from build123d import *

# Parameters (mm, degrees)
SKETCH_W        = 4.72
SKETCH_H        = 5.2
PAD_DEPTH       = 18.3
POCKET_DEPTH    = 38.001
SKETCH002_R     = 1.5
POCKET001_DEPTH = 6
PAD001_DEPTH    = 13
SKETCH004_W     = 2
SKETCH004_H     = 0.982872
POCKET002_DEPTH = 38.001
POCKET003_DEPTH = 51.701
FILLET_R        = 1
CHAMFER_SIZE    = 0.5
FILLET001_R     = 1


with BuildPart() as part:
    # Sketch → Pad (new body)
    with BuildSketch(Plane.XY):
        Polygon((-19, 22), (-19, -22), (19, -22), (19, 22), (17, 22), (17, 29.7), (6, 29.7), (6, 22), (-6, 22), (-6, 29.7), (-17, 29.7), (-17, 22), align=None)
        with Locations((-12.41, 24.6)):
            Rectangle(SKETCH_W, SKETCH_H, mode=Mode.SUBTRACT)
        with Locations((12.41, 24.6)):
            Rectangle(SKETCH_W, SKETCH_H, mode=Mode.SUBTRACT)
    extrude(amount=PAD_DEPTH)

    # Sketch001 (on Face3 of Pad) → Pocket (cut, through all)
    with BuildSketch(Plane.YZ.offset(19)):
        with BuildLine():
            Line((29.7, 11.3), (29.7, 0))
            Line((29.7, 0), (-21.3, 0))
            ThreePointArc((3.7, 11.3), (-10.017598, 8.343801), (-21.3, 0))
            Line((29.7, 11.3), (3.7, 11.3))
        make_face()
    extrude(amount=-POCKET_DEPTH, mode=Mode.SUBTRACT)

    # Sketch002 (on Face5 of Pocket) → Pocket001 (cut)
    with BuildSketch(Plane.XZ.offset(22)):
        with Locations((-15.844609, 11.767382)):
            Circle(SKETCH002_R)
        with Locations((15.754541, 11.777902)):
            Circle(SKETCH002_R)
    extrude(amount=-POCKET001_DEPTH, mode=Mode.SUBTRACT)

    # Sketch003 (on Face1 of Pocket001) → Pad001 (join)
    with BuildSketch(Plane(origin=(-19, 0, 0), x_dir=(0, -1, 0), z_dir=(-1, 0, 0))):
        with BuildLine():
            Line((20, 18.3), (1.881002, 18.3))
            ThreePointArc((1.881002, 18.3), (10.537629, 21.219302), (15.5, 28.88966))
            Line((20, 28.88966), (15.5, 28.88966))
            Line((20, 18.3), (20, 28.88966))
        make_face()
    pad001 = extrude(amount=-PAD001_DEPTH)

    # Mirrored: Pad001 across YZ
    add(pad001.mirror(Plane.YZ))

    # Sketch004 (on Face5 of Mirrored) → Pocket002 (cut, through all)
    with BuildSketch(Plane(origin=(-19, 0, 0), x_dir=(0, -1, 0), z_dir=(-1, 0, 0))):
        with Locations((21, 17.808564)):
            Rectangle(SKETCH004_W, SKETCH004_H)
    extrude(amount=-POCKET002_DEPTH, mode=Mode.SUBTRACT)

    # Sketch005 (on Face23 of Pocket002) → Pocket003 (cut, through all)
    with BuildSketch(Plane.XZ.offset(22)):
        with BuildLine():
            add(Edge.make_bspline(
                [(-19.030813, 9.913328), (-19.030294, 8.01238), (-17.308198, 7.207429)],
                knots=[1.082896, 1.082896, 1.082896, 2.216203, 2.216203, 2.216203], degree=2, weights=[1, 0.843702, 1]))
            Line((-17.308198, 7.207429), (-3.577259, 0.790051))
            add(Edge.make_bspline(
                [(-3.577259, 0.790051), (-1.968517, 0.037468), (-0.192474, 0.03938)],
                knots=[2.215888, 2.215888, 2.215888, 2.654527, 2.654527, 2.654527], degree=2, weights=[1, 0.976046, 1]))
            Line((-0.192474, 0.03938), (0.111534, 0.039482))
            add(Edge.make_bspline(
                [(0.111534, 0.039482), (1.887576, 0.038752), (3.495769, 0.792404)],
                knots=[2.653039, 2.653039, 2.653039, 3.091677, 3.091677, 3.091677], degree=2, weights=[1, 0.976046, 1]))
            Line((3.495769, 0.792404), (17.222042, 7.218925))
            add(Edge.make_bspline(
                [(17.222042, 7.218925), (18.943553, 8.025023), (18.94269, 9.92597)],
                knots=[3.091363, 3.091363, 3.091363, 4.22467, 4.22467, 4.22467], degree=2, weights=[1, 0.843702, 1]))
            Line((18.94269, 9.92597), (19.755945, 10.17424))
            Line((19.755945, 10.17424), (19.755945, -1.191288))
            Line((19.755945, -1.191288), (-20.023405, -1.191288))
            Line((-20.023405, -1.191288), (-20.023405, 9.913328))
            Line((-20.023405, 9.913328), (-19.030813, 9.913328))
        make_face()
    extrude(amount=-POCKET003_DEPTH, mode=Mode.SUBTRACT)

    # Fillet
    fillet_edges = [part.edges().sort_by_distance(p)[0] for p in [
        (19, 22, 14.8),
        (17, 29.7, 14.8),
        (6, 29.7, 14.8),
        (-6, 29.7, 14.8),
        (-17, 29.7, 14.8),
        (-19, 22, 14.8),
    ]]
    fillet(fillet_edges, radius=FILLET_R)

    # Chamfer
    chamfer_edges = [part.edges().sort_by_distance(p)[0] for p in [
        (12.41, 22, 11.3),
        (10.05, 24.6, 11.3),
        (12.41, 27.2, 11.3),
        (14.77, 24.6, 11.3),
        (-10.05, 24.6, 11.3),
        (-12.41, 22, 11.3),
        (-14.77, 24.6, 11.3),
        (-12.41, 27.2, 11.3),
    ]]
    chamfer(chamfer_edges, length=CHAMFER_SIZE)

    # Fillet001
    fillet001_edges = [part.edges().sort_by_distance(p)[0] for p in [
        (-12.5, -15.5, 28.88966),
        (12.5, -15.5, 28.88966),
    ]]
    fillet(fillet001_edges, radius=FILLET001_R)


solid = part.part
Read the model definition and answer for the solid it produces. Units are mm, in the model's axes. A direction names the side the tool comes from. Round coordinates to 2 decimals unless told otherwise and drop trailing zeros. Write each loop counter-clockwise with the first axis right and the second up, starting at its lowest first coordinate (ties: lowest second). Pieces come first, ordered by that corner, then holes. Notation, with made-up numbers: M 15.5,-21 L 71.5,-21 A17 ccw 71.5,-14 Z; hole C 22,-28 d10. An arc over 180 degrees is marked long. Use a Markdown table: item, result.
1) A tool of negligible diameter and unlimited length cuts with its end or side. For faces 4 (the flat face through (6, 25, 15)), 5 (the flat face through (-12, 27.2, 15)), 6 (the flat face through (-6, -15, 22)), from which of +Z, -Z, +X, -X, +Y, -Y can it reach the whole face along a straight path? Write none if from no direction.
Answers follow:
| item | result |
|---|---|
| face 4 | +Z, -Z, +Y |
| face 5 | +Z, -Z |
| face 6 | +Z, +Y, -Y |
2) The part is cut by section C-C (x = -12). Write down the section's boundary in (y, z).
Answers follow:
| item | result |
|---|---|
| outline | M -22,4.73 L -16.17,4.73 A33.3 cw 3.7,11.3 L 21.5,11.3 L 22,11.8 L 22,18.3 L -2.17,18.3 A13.87 cw -15.31,28.18 A1 ccw -16.26,28.89 L -20,28.89 L -20,17.32 L -22,17.32 Z; M 27.2,11.8 L 27.7,11.3 L 29.7,11.3 L 29.7,18.3 L 27.2,18.3 Z |
3) The part is cut by section A-A (y = 25). Write down the section's boundary in (x, z), plus the area to 3 significant figures.
Answers follow:
| item | result |
|---|---|
| outline | M -17,11.3 L -15.27,11.3 L -14.77,11.8 L -14.77,18.3 L -17,18.3 Z; M -10.05,11.8 L -9.55,11.3 L -6,11.3 L -6,18.3 L -10.05,18.3 Z; M 6,11.3 L 9.55,11.3 L 10.05,11.8 L 10.05,18.3 L 6,18.3 Z; M 14.77,11.8 L 15.27,11.3 L 17,11.3 L 17,18.3 L 14.77,18.3 Z |
| area | 87.4 mm2 |
4) Straight lines are drawn through the part: line 1 along X through (y, z) = (-7.5, 19.25); line 2 along Z through (x, y) = (3, -4.5); line 3 along Z through (x, y) = (8, 19). For each, find the intervals that lie inside material, in ascending order. Write a range as [from, to].
Answers follow:
| item | result |
|---|---|
| line 1 | x = [-19, -6], [6, 19] |
| line 2 | z = [10.27, 18.3] |
| line 3 | z = [11.3, 18.3] |
5) The part is cut by section B-B (z = 16.25). Write down the section's boundary in (x, y), plus the area to 3 significant figures.
Answers follow:
| item | result |
|---|---|
| outline | M -19,-22 L 19,-22 L 19,21 A1 ccw 18,22 L 17,22 L 17,28.7 A1 ccw 16,29.7 L 7,29.7 A1 ccw 6,28.7 L 6,22 L -6,22 L -6,28.7 A1 ccw -7,29.7 L -16,29.7 A1 ccw -17,28.7 L -17,22 L -18,22 A1 ccw -19,21 Z; hole M -14.77,22 L -10.05,22 L -10.05,27.2 L -14.77,27.2 Z; hole M 10.05,22 L 14.77,22 L 14.77,27.2 L 10.05,27.2 Z |
| area | 1,790 mm2 |
6) For a pull along X with two mould halves and no side action, classify faces 1 (the flat face through (12, 22, 15)), 2 (the flat face through (-12.065, -19.372, 4.757)), 3 (the flat face through (-13, -18, 28.89)) as pulls with the +X half, pulls with the -X half, needs draft (parallel to the pull), parting line crosses it, or undercut.
Answers follow:
| item | result |
|---|---|
| face 1 | undercut |
| face 2 | pulls with the -X half |
| face 3 | needs draft |
7) Flat-ended cylindrical pins translate along their axes: pin 1 (4 mm diameter, centred on y = 26, z = 14, fed in from -X); pin 2 (4 mm diameter, centred on x = 11, y = -10.5, fed in from -Z); pin 3 (8 mm diameter, centred on x = 7, y = -14.5, fed in from -Z). Find the tip coordinate at first contact, or state that the pin passes through.
Answers follow:
| item | result |
|---|---|
| pin 1 | stops at x = -17 |
| pin 2 | stops at z = 7.09 |
| pin 3 | stops at z = 2.82 |
8) The part is cut by section D-D (z = 20.25). Write down the section's boundary in (x, y), plus the area to 3 significant figures.
Answers follow:
| item | result |
|---|---|
| outline | M -19,-20 L -6,-20 L -6,-9.12 L -19,-9.12 Z; M 6,-20 L 19,-20 L 19,-9.12 L 6,-9.12 Z |
| area | 283 mm2 |
